Drawing for the job (mm, zero at the part's lowest x, y, z). A direction names the side the tool comes from. Round coordinates to 2 decimals unless told otherwise and drop trailing zeros. Loops run counter-clockwise (first coordinate to the right, second up) from the corner with the lowest first, then second, coordinate; pieces in that order, holes last. Notation, with made-up numbers: M 34.25,68.25 L 81.25,68.25 A36 cw 81.25,106.25 Z; hole C 85.5,88 d4. An arc over 180 degrees is marked long. Answer in a Markdown table with one row per item.
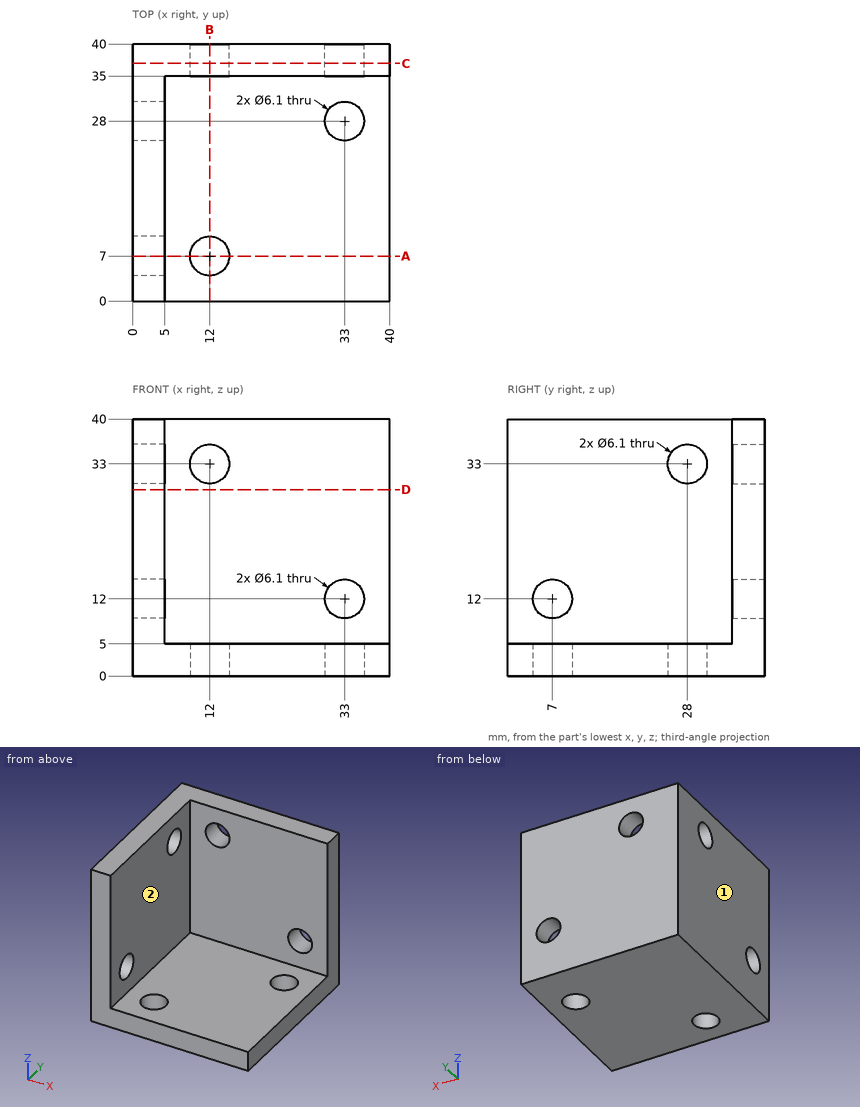
1. Saw through at B-B (x = 12). Write the cut outline in (y, z), and give its area (3 significant figures).
Verdict:
| item | result |
|---|---|
| outline | M 0,0 L 3.95,0 L 3.95,5 L 0,5 Z; M 10.05,0 L 40,0 L 40,29.95 L 35,29.95 L 35,5 L 10.05,5 Z; M 35,36.05 L 40,36.05 L 40,40 L 35,40 Z |
| area | 314 mm² |
2. Saw through at D-D (z = 29). Write the cut outline in (x, y).
Verdict:
| item | result |
|---|---|
| outline | M 0,0 L 5,0 L 5,35 L 40,35 L 40,40 L 0,40 Z |
3. Saw through at A-A (y = 7). Write the cut outline in (x, z), and give its area (3 significant figures).
Verdict:
| item | result |
|---|---|
| outline | M 0,0 L 8.95,0 L 8.95,5 L 5,5 L 5,8.95 L 0,8.95 Z; M 0,15.05 L 5,15.05 L 5,40 L 0,40 Z; M 15.05,0 L 40,0 L 40,5 L 15.05,5 Z |
| area | 314 mm² |
4. Wall check: probe 1 along Z at (x, y) = (1.8, 28); probe 2 along Y at (x, z) = (2, 12); probe 3 along Y at (x, z) = (10, 13.5). Give the ranges that are in metal, low to high.
Verdict:
| item | result |
|---|---|
| probe 1 | z = 0 to 29.95, 36.05 to 40 |
| probe 2 | y = 0 to 3.95, 10.05 to 40 |
| probe 3 | y = 35 to 40 |
5. Saw through at C-C (y = 37). Write the cut outline in (x, z), and give its area (3 significant figures).
Verdict:
| item | result |
|---|---|
| outline | M 0,0 L 40,0 L 40,40 L 0,40 Z; hole C 12,33 d6.1; hole C 33,12 d6.1 |
| area | 1,540 mm² |
6. Tool access for the marked faces 1 and 2: list every direction of +Z, -Z, +X, -X, +Y, -Y with a clear straight run to the whole face (end or side of a thin tool).
Verdict:
| item | result |
|---|---|
| face 1 | +Z, -Z, -X, +Y, -Y |
| face 2 | +Z, +X, -Y |
7. Pin check, flat tips, straight feed: pin 1 (8 mm diameter, centred on x = 33, y = 28, fed in from +Z); pin 2 (10.5 mm diameter, centred on y = 22.5, z = 17.5, fed in from +X); pin 3 (3 mm diameter, centred on x = 17.5, z = 17, fed in from -Y). Stop position of each tip, or through.
Verdict:
| item | result |
|---|---|
| pin 1 | stops at z = 5 |
| pin 2 | stops at x = 5 |
| pin 3 | stops at y = 35 |
